The listing builds one solid part. Answer for the finished solid, in the listing's coordinates (mm). A direction names the side the tool comes from. Give positions to 0.01 mm unless a question says otherwise; leave off trailing zeros. Loops run counter-clockwise (first coordinate to the right, second up) from the corner with the lowest first, then second, coordinate; pieces in that order, holes last. Notation, with made-up numbers: (29, -33.5) - (78, -33.5) arc R22 cw to (78, -21.5) - close; hole circle Ø11 at (54.25, 14). An arc over 180 degrees is marked (long way). Answer in a Markdown table with one row per item. Add a question column.
Solid Edge part; units mm, degrees
sketch "Sketch1" plane through (0, 0, 0) normal (0, -1, 0) x (1, 0, 0)
  line L0 (-16, -3.85) -> (16, -3.85)
  line L1 (16, -3.85) -> (16, 3.85)
  line L2 (16, 3.85) -> (-16, 3.85)
  line L3 (-16, 3.85) -> (-16, -3.85)
extrude "Protrusion1" add sketch "Sketch1" against normal blind 1.5
sketch "Sketch2" plane through (0, 1.5, 0) normal (0, 1, 0) x (-1, 0, 0)
  line L0 (7.9, 3.85) -> (-7.9, 3.85)
  line L1 (-7.9, 3.85) -> (-7.9, 0.75)
  line L2 (-7.9, 0.75) -> (7.9, 0.75)
  line L3 (7.9, 0.75) -> (7.9, 3.85)
extrude "ExtrudedProtrusion_2" add sketch "Sketch2" along normal blind 8
sketch "Sketch3" plane through (0, 5.5, 0.75) normal (0, 0, -1) x (0, 1, 0)
  line L0 (2.4, -6.45) -> (-4, -6.45)
  line L1 (-4, -6.45) -> (-4, -4.3)
  line L2 (-2.6, -4.3) -> (-4, -4.3)
  line L3 (-2.6, -3.2) -> (-2.6, -4.3)
  line L4 (-2.6, -3.2) -> (-4, -3.2)
  line L5 (-4, -3.2) -> (-4, -0.55)
  line L6 (-2.6, -0.55) -> (-4, -0.55)
  line L7 (-2.6, 0.55) -> (-2.6, -0.55)
  line L8 (-2.6, 0.55) -> (-4, 0.55)
  line L9 (-4, 0.55) -> (-4, 3.2)
  line L10 (-2.6, 3.2) -> (-4, 3.2)
  line L11 (-2.6, 4.3) -> (-2.6, 3.2)
  line L12 (-2.6, 4.3) -> (-4, 4.3)
  line L13 (-4, 4.3) -> (-4, 6.45)
  line L14 (-4, 6.45) -> (2.4, 6.45)
  line L15 (2.4, 6.45) -> (2.4, -6.45)
  circle A0 centre (0, 0) radius 1.4
  circle A1 centre (0, 0) radius 0.95
extrude "ExtrudedCutout_1" cut sketch "Sketch3" against normal blind 1.8
sketch "Sketch4" plane through (0, 4.7, 2.55) normal (0, 0, -1) x (0, 1, 0)
  circle A0 centre (0.8, 4) radius 1.5
  circle A1 centre (0.8, -4) radius 1.5
extrude "ExtrudedCutout_2" cut sketch "Sketch4" against normal blind 2.4
sketch "Sketch5" plane through (0, 4.75, 3.85) normal (0, 0, 1) x (1, 0, 0)
  circle A0 centre (-4, 0.75) radius 2.4
  circle A1 centre (4, 0.75) radius 2.4
extrude "ExtrudedProtrusion_3" add sketch "Sketch5" along normal blind 1.8
sketch "Sketch6" plane through (0, 0, 0) normal (0, -1, 0) x (1, 0, 0)
  circle A0 centre (-12, 0) radius 2.4
  circle A1 centre (-4, 0) radius 2.4
  circle A2 centre (4, 0) radius 2.4
  circle A3 centre (12, 0) radius 2.4
  circle A4 centre (-12, 0) radius 1.6
  circle A5 centre (-4, 0) radius 1.6
  circle A6 centre (4, 0) radius 1.6
  circle A7 centre (12, 0) radius 1.6
extrude "ExtrudedProtrusion_4" add sketch "Sketch6" along normal blind 1.8
(1) Find the intervals of material crossed by line 1 along X through (y, z) = (5.5, 2.75); line 2 along Z through (x, y) = (-4, -0.5); line 3 along Y through (x, z) = (-3.5, 2), in increasing order. Write a range as [from, to].
(2) The mould has two halves that part along Z. Classify faces 6 (the face through (-1.71, -0.89, -0.72)), 7 (the face through (-4.3, 2, 2)), 8 (the face through (10.4, -0.89, -0.07)): pulls with the +Z half, pulls with the -Z half, needs draft (parallel to the pull), parting line crosses it, or undercut.
(3) A cutting plane is placed at B-B on x = 0. Determine the outline of the cut face in (y, z).
(4) A cutting plane is placed at D-D on z = -3. Determine the outline of the cut face in (x, y).
(5) A cutting plane is placed at C-C on z = 5.25. Determine the outline of the cut face in (x, y), plus the area to 3 significant figures.
(6) A tool of negligible diameter and unlimited length cuts with its end or side. For faces 1 (the face through (-7.9, 5, 2)), 2 (the face through (-0.55, 2, 2)), 3 (the face through (4, 2, 0.75)), 4 (the face through (-2.71, 3.476, 4.737)), 5 (the face through (12, 0, 0)), from which of +Z, -Z, +X, -X, +Y, -Y can it reach the whole face along a straight path? Write none if from no direction.
(7) Given pin 1 Ø3.5 at (x, y) = (-4, 5.5) entering from -Z; pin 2 Ø1.1 at (y, z) = (2, 2) entering from +X; pin 3 Ø4 at (x, y) = (1, 5.5) entering from -Z; pin 4 Ø2 at (x, z) = (5.5, -2.5) entering from +Y, each flat-ended and moving along its own axis, determine where each tip first touches the part or whether it passes through.
(8) A cutting plane is placed at A-A on y = 2.5. Determine the outline of the cut face in (x, z).
Evaluation:
| question | item | result |
|---|---|---|
| 1 | line 1 | x = [-7.9, -5.5], [-2.5, 2.5], [5.5, 7.9] |
| 1 | line 2 | z = [-2.4, -1.6], [1.6, 2.4] |
| 1 | line 3 | y = [-1.8, 2.9], [7.9, 9.5] |
| 2 | face 6 | parting line crosses it |
| 2 | face 7 | needs draft |
| 2 | face 8 | undercut |
| 3 | outline | (0, -3.85) - (1.5, -3.85) - (1.5, 0.75) - (2.9, 0.75) - (2.9, 2.55) - (4.1, 2.55) - (4.1, 0.75) - (4.55, 0.75) - (4.55, 2.55) - (6.45, 2.55) - (6.45, 0.75) - (6.9, 0.75) - (6.9, 2.55) - (7.9, 2.55) - (7.9, 0.75) - (9.5, 0.75) - (9.5, 3.85) - (0, 3.85) - close |
| 4 | outline | (-16, 0) - (16, 0) - (16, 1.5) - (-16, 1.5) - close |
| 5 | outline | circle Ø4.8 at (-4, 5.5); circle Ø4.8 at (4, 5.5) |
| 5 | area | 36.2 mm² |
| 6 | face 1 | +Z, -Z, -X, +Y |
| 6 | face 2 | -Z |
| 6 | face 3 | -Z, +X, -X, +Y |
| 6 | face 4 | +Z |
| 6 | face 5 | -Y |
| 7 | pin 1 | stops at z = 2.55 |
| 7 | pin 2 | stops at x = 16 |
| 7 | pin 3 | stops at z = 0.75 |
| 7 | pin 4 | stops at y = 1.5 |
| 8 | outline | (-7.9, 0.75) - (-6.45, 0.75) - (-6.45, 2.55) - (-4.3, 2.55) - (-4.3, 0.75) - (-3.2, 0.75) - (-3.2, 2.55) - (-0.55, 2.55) - (-0.55, 0.75) - (0.55, 0.75) - (0.55, 2.55) - (3.2, 2.55) - (3.2, 0.75) - (4.3, 0.75) - (4.3, 2.55) - (6.45, 2.55) - (6.45, 0.75) - (7.9, 0.75) - (7.9, 3.85) - (-7.9, 3.85) - close |
